Here's how the part is built. I have some questions about the finished solid (model axes, mm). Give positions to 0.01 mm unless a question says otherwise; leave off trailing zeros. Order: outer loops, then holes, each group sorted by start corner. A loop starts at its lowest first (then second) coordinate and runs counter-clockwise, first axis right, second up. Notation, with made-up numbers: M 59.5,13.5 L 105.5,13.5 A30 ccw 105.5,40.5 Z; hole C -25,-31 d2. An arc over 180 degrees is marked long. Use one line per item in the form item = value.
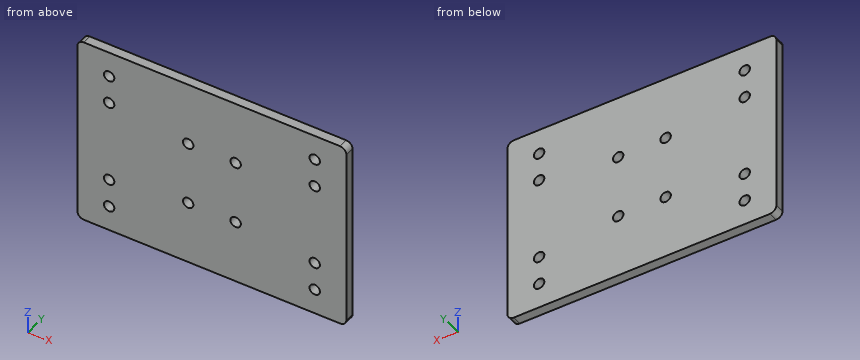
from build123d import *

# Parameters (mm, degrees)
SKETCH_1_W          = 85
SKETCH_1_H          = 60
EXTRUDE_1_DEPTH     = 3
SKETCH_2_R          = 1.65
CUT_EXTRUDE_1_DEPTH = 3
SKETCH_3_R          = 1.65
CUT_EXTRUDE_2_DEPTH = 100
FILLET_1_R          = 2


with BuildPart() as part:
    # 草图1 → 凸台-拉伸1 (new body)
    with BuildSketch(Plane(origin=(0, 0, 0), x_dir=(1, 0, 0), z_dir=(0, 1, 0))):
        Rectangle(SKETCH_1_W, SKETCH_1_H)
    extrude(amount=EXTRUDE_1_DEPTH)

    # 草图2 → 切除-拉伸1 (cut)
    with BuildSketch(Plane(origin=(0, 3, 0), x_dir=(1, 0, 0), z_dir=(0, 1, 0))):
        with Locations(Location((7.5, 10, 0), (0, 0, 270))):
            Circle(SKETCH_2_R)
        with Locations(Location((-7.5, 10, 0), (0, 0, 270))):
            Circle(SKETCH_2_R)
        with Locations(Location((-7.5, -10, 0), (0, 0, 270))):
            Circle(SKETCH_2_R)
        with Locations(Location((7.5, -10, 0), (0, 0, 270))):
            Circle(SKETCH_2_R)
    extrude(amount=-CUT_EXTRUDE_1_DEPTH, mode=Mode.SUBTRACT)

    # 草图3 → 切除-拉伸2 (cut)
    with BuildSketch(Plane(origin=(0, 3, 0), x_dir=(1, 0, 0), z_dir=(0, 1, 0))):
        with Locations(Location((32.5, 13, 0), (0, 0, 270))):
            Circle(SKETCH_3_R)
        with Locations(Location((32.5, 22, 0), (0, 0, 270))):
            Circle(SKETCH_3_R)
        with Locations(Location((32.5, -13, 0), (0, 0, 90))):
            Circle(SKETCH_3_R)
        with Locations(Location((32.5, -22, 0), (0, 0, 90))):
            Circle(SKETCH_3_R)
    cut_extrude_2 = extrude(amount=-CUT_EXTRUDE_2_DEPTH, mode=Mode.SUBTRACT)

    # 镜向1: 切除-拉伸2 across plane
    add(cut_extrude_2.mirror(Plane(origin=(0, 0, 0), x_dir=(0, 0, 1), z_dir=(1, 0, 0))), mode=Mode.SUBTRACT)

    # 圆角1
    fillet_1_edges = [part.edges().sort_by_distance(p)[0] for p in [
        (42.5, 1.5, 30),
        (-42.5, 1.5, 30),
        (-42.5, 1.5, -30),
        (42.5, 1.5, -30),
    ]]
    fillet(fillet_1_edges, radius=FILLET_1_R)


solid = part.part
Q1. I want a section at D-D on x = -32.5. Write out the boundary of the cut face in (y, z), then the cut area to 3 significant figures.
Found:
outline = M 0,-30 L 3,-30 L 3,-23.65 L 0,-23.65 Z; M 0,-20.35 L 3,-20.35 L 3,-14.65 L 0,-14.65 Z; M 0,-11.35 L 3,-11.35 L 3,11.35 L 0,11.35 Z; M 0,14.65 L 3,14.65 L 3,20.35 L 0,20.35 Z; M 0,23.65 L 3,23.65 L 3,30 L 0,30 Z
area = 140 mm²
Q2. I want a section at A-A on z = 22. Write out the boundary of the cut face in (x, y).
Found:
outline = M -42.5,0 L -34.15,0 L -34.15,3 L -42.5,3 Z; M -30.85,0 L 30.85,0 L 30.85,3 L -30.85,3 Z; M 34.15,0 L 42.5,0 L 42.5,3 L 34.15,3 Z
Q3. I want a section at C-C on y = 2.5. State how many separate pieces and enclosed holes the cut face has, then the cut area to 3 significant figures.
Found:
separate_pieces = 1
enclosed_holes = 12
area = 4,990 mm²
Q4. I want a section at B-B on x = -7.5. Write out the boundary of the cut face in (y, z), then the cut area to 3 significant figures.
Found:
outline = M 0,-30 L 3,-30 L 3,-11.65 L 0,-11.65 Z; M 0,-8.35 L 3,-8.35 L 3,8.35 L 0,8.35 Z; M 0,11.65 L 3,11.65 L 3,30 L 0,30 Z
area = 160 mm²
Q5. I need wall thicknesses on L1, parallel to X at y = 0.8, z = -13; L2, parallel to X at y = 0.7, z = -10; L3, parallel to Z at x = 32, y = 0.6. Which ranges of each line are inside material? Lowest first, please.
Found:
L1 = -42.5 to -34.15, -30.85 to 30.85, 34.15 to 42.5
L2 = -42.5 to -9.15, -5.85 to 5.85, 9.15 to 42.5
L3 = -30 to -23.57, -20.43 to -14.57, -11.43 to 11.43, 14.57 to 20.43, 23.57 to 30
